Read the model definition and answer for the solid it produces. Units are mm, in the model's axes. A direction names the side the tool comes from. Coordinates: 2 decimals unless noted, no trailing zeros. Loops run counter-clockwise (first coordinate to the right, second up) from the corner with the lowest first, then second, coordinate; pieces in that order, holes last. Notation, with made-up numbers: (-37, 23) -> (-4, 23) arc R34 cw to (-4, 57) -> close; hole circle Ø2 at (-29, 49.5). An arc over 180 degrees is marked (long way). Answer in a Markdown table with one row per item.
```python
from build123d import *

# Parameters (mm, degrees)
SKETCH_1_R          = 1
EXTRUDE_1_DEPTH     = 5.5
SKETCH_2_R          = 2
EXTRUDE_2_DEPTH     = 2
CUT_EXTRUDE_1_DEPTH = 1


with BuildPart() as part:
    # 草图1 → 凸台-拉伸1 (new body)
    with BuildSketch(Plane.XY):
        Circle(SKETCH_1_R)
    extrude(amount=EXTRUDE_1_DEPTH)

    # 草图2 → 凸台-拉伸2 (add)
    with BuildSketch(Plane(origin=(0, 0, 0), x_dir=(-1, 0, 0), z_dir=(0, 0, -1))):
        Circle(SKETCH_2_R)
    extrude(amount=EXTRUDE_2_DEPTH)

    # 草图3 → 切除-拉伸1 (cut)
    with BuildSketch(Plane(origin=(0, 0, -2), x_dir=(-1, 0, 0), z_dir=(0, 0, -1))):
        Polygon((1, 0), (0.5, 0.866025404), (-0.5, 0.866025404), (-1, 0), (-0.5, -0.866025404), (0.5, -0.866025404), align=None)
    extrude(amount=-CUT_EXTRUDE_1_DEPTH, mode=Mode.SUBTRACT)


solid = part.part
```
1. A cutting plane is placed at C-C on z = 3. Give the vertices of the cut face in (x, y).
A:
| item | result |
|---|---|
| outline | circle Ø2 at (0, 0) |
2. The mould has two halves that part along Y. Classify faces 4 (the cylindrical face through (0, -1, 3)), 5 (the flat face through (0, 0, 5.5)), 6 (the flat face through (0.746, 0.439, -1.507)): pulls with the +Y half, pulls with the -Y half, needs draft (parallel to the pull), parting line crosses it, or undercut.
A:
| item | result |
|---|---|
| face 4 | parting line crosses it |
| face 5 | needs draft |
| face 6 | undercut |
3. A tool of negligible diameter and unlimited length cuts with its end or side. For faces 1 (the flat face through (0, 0.866, -1.5)), 2 (the cylindrical face through (0, -2, -1)), 3 (the flat face through (-1, -1, 0)), from which of +Z, -Z, +X, -X, +Y, -Y can it reach the whole face along a straight path? Write none if from no direction.
A:
| item | result |
|---|---|
| face 1 | -Z |
| face 2 | +Z, -Z |
| face 3 | +Z |
4. A cutting plane is placed at A-A on x = 0. Give the vertices of the cut face in (y, z).
A:
| item | result |
|---|---|
| outline | (-2, -2) -> (-0.87, -2) -> (-0.87, -1) -> (0.87, -1) -> (0.87, -2) -> (2, -2) -> (2, 0) -> (1, 0) -> (1, 5.5) -> (-1, 5.5) -> (-1, 0) -> (-2, 0) -> close |
5. A cutting plane is placed at B-B on y = -0.5. Give the vertices of the cut face in (x, z).
A:
| item | result |
|---|---|
| outline | (-1.94, -2) -> (-0.71, -2) -> (-0.71, -1) -> (0.71, -1) -> (0.71, -2) -> (1.94, -2) -> (1.94, 0) -> (0.87, 0) -> (0.87, 5.5) -> (-0.87, 5.5) -> (-0.87, 0) -> (-1.94, 0) -> close |
6. Find the intervals of material crossed by probe 1 along Z at (x, y) = (-0.45, -0.25); probe 2 along Z at (x, y) = (1.25, -0.95); probe 3 along Y at (x, z) = (-0.85, -1.5), in increasing order.
A:
| item | result |
|---|---|
| probe 1 | z = -1 to 5.5 |
| probe 2 | z = -2 to 0 |
| probe 3 | y = -1.81 to -0.26, 0.26 to 1.81 |
7. A cutting plane is placed at D-D on x = 1.35. Give the vertices of the cut face in (y, z).
A:
| item | result |
|---|---|
| outline | (-1.48, -2) -> (1.48, -2) -> (1.48, 0) -> (-1.48, 0) -> close |
